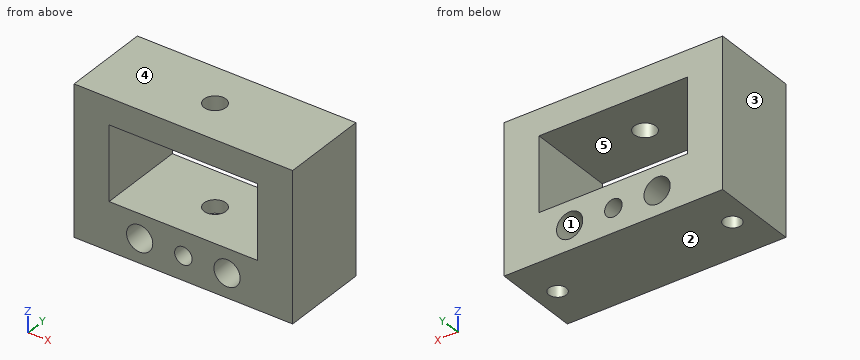
from build123d import *

# Parameters (mm, degrees)
SKETCH1_W                = 50
SKETCH1_H                = 20
BOSS_EXTRUDE1_DEPTH      = 11
SKETCH2_R                = 2
CUT_EXTRUDE1_DEPTH       = 11
SKETCH3_R                = 2
CUT_EXTRUDE2_DEPTH       = 21
SKETCH4_R                = 3
CUT_EXTRUDE3_DEPTH       = 21
SKETCH5_W                = 8
SKETCH5_H                = 20
BOSS_EXTRUDE2_DEPTH      = 22
SKETCH13_R               = 2.5
CUT_EXTRUDE6_DEPTH       = 3
SKETCH14_W               = 50
SKETCH14_H               = 20
BOSS_EXTRUDE4_DEPTH      = 1
BOSS_EXTRUDE4_DEPTH_BACK = 5
SKETCH15_R               = 2.5
CUT_EXTRUDE7_DEPTH       = 6
SKETCH18_R               = 2
CUT_EXTRUDE8_DEPTH       = 13


with BuildPart() as part:
    # Sketch1 → Boss-Extrude1 (new body)
    with BuildSketch(Plane.XY):
        Rectangle(SKETCH1_W, SKETCH1_H)
    extrude(amount=BOSS_EXTRUDE1_DEPTH)

    # Sketch2 → Cut-Extrude1 (cut)
    with BuildSketch(Plane(origin=(0, 0, 0), x_dir=(-1, 0, 0), z_dir=(0, 0, -1))):
        with Locations((-20, 0)):
            Circle(SKETCH2_R)
        with Locations((20, 0)):
            Circle(SKETCH2_R)
    extrude(amount=-CUT_EXTRUDE1_DEPTH, mode=Mode.SUBTRACT)

    # Sketch3 → Cut-Extrude2 (cut, through all)
    with BuildSketch(Plane.XZ.offset(10)):
        with Locations((0, 5.5)):
            Circle(SKETCH3_R)
    extrude(amount=-CUT_EXTRUDE2_DEPTH, mode=Mode.SUBTRACT)

    # Sketch4 → Cut-Extrude3 (cut, through all)
    with BuildSketch(Plane.XZ.offset(10)):
        with Locations((-10, 5.5)):
            Circle(SKETCH4_R)
        with Locations((10, 5.5)):
            Circle(SKETCH4_R)
    extrude(amount=-CUT_EXTRUDE3_DEPTH, mode=Mode.SUBTRACT)

    # Sketch5 → Boss-Extrude2 (add)
    with BuildSketch(Plane.XY.offset(11)):
        with Locations((-21, 0)):
            Rectangle(SKETCH5_W, SKETCH5_H)
        with Locations((21, 0)):
            Rectangle(SKETCH5_W, SKETCH5_H)
    extrude(amount=BOSS_EXTRUDE2_DEPTH)

    # Sketch13 → Cut-Extrude6 (cut)
    with BuildSketch(Plane.XY.offset(11)):
        Circle(SKETCH13_R)
    extrude(amount=-CUT_EXTRUDE6_DEPTH, mode=Mode.SUBTRACT)

    # Sketch14 → Boss-Extrude4 (add, two sides)
    with BuildSketch(Plane.XY.offset(33)) as boss_extrude4_sk:
        Rectangle(SKETCH14_W, SKETCH14_H)
    extrude(amount=BOSS_EXTRUDE4_DEPTH)
    extrude(boss_extrude4_sk.sketch, amount=-BOSS_EXTRUDE4_DEPTH_BACK)

    # Sketch15 → Cut-Extrude7 (cut)
    with BuildSketch(Plane.XY.offset(34)):
        Circle(SKETCH15_R)
    extrude(amount=-CUT_EXTRUDE7_DEPTH, mode=Mode.SUBTRACT)

    # Sketch18 → Cut-Extrude8 (cut)
    with BuildSketch(Plane(origin=(0, 0, 11), x_dir=(-1, 0, 0), z_dir=(0, 0, -1))):
        with Locations((-20, 0)):
            Circle(SKETCH18_R)
        with Locations((20, 0)):
            Circle(SKETCH18_R)
    extrude(amount=-CUT_EXTRUDE8_DEPTH, mode=Mode.SUBTRACT)


solid = part.part
Build history of the part. All positions in model axes, mm. Face numbers are marked on the shaded views. A direction names the side the tool comes from. Give positions to 0.01 mm unless a question says otherwise; leave off trailing zeros. Loops run counter-clockwise (first coordinate to the right, second up) from the corner with the lowest first, then second, coordinate; pieces in that order, holes last. Notation, with made-up numbers: (21.25, -9) -> (68.25, -9) arc R28 ccw to (68.25, 29) -> close; hole circle Ø8 at (41.5, 39.25). An arc over 180 degrees is marked (long way). Answer in a Markdown table with one row per item.
Item 1: Mould opens along X. For the marked faces 1, 2 and 3 say: pulls with the +X half, pulls with the -X half, needs draft (parallel to the pull), parting line crosses it, or undercut.
Findings below:
| item | result |
|---|---|
| face 1 | undercut |
| face 2 | needs draft |
| face 3 | pulls with the -X half |
Item 2: Slice it at B-B on x = 10. Write the cut outline in (y, z).
Findings below:
| item | result |
|---|---|
| outline | (-10, 0) -> (10, 0) -> (10, 2.5) -> (-10, 2.5) -> close; (-10, 8.5) -> (10, 8.5) -> (10, 11) -> (-10, 11) -> close; (-10, 28) -> (10, 28) -> (10, 34) -> (-10, 34) -> close |
Item 3: Slice it at A-A on z = 22.5. Write the cut outline in (x, y).
Findings below:
| item | result |
|---|---|
| outline | (-25, -10) -> (-17, -10) -> (-17, 10) -> (-25, 10) -> close; (17, -10) -> (25, -10) -> (25, 10) -> (17, 10) -> close; hole circle Ø4 at (-20, 0); hole circle Ø4 at (20, 0) |
Item 4: Slice it at C-C on z = 5.5. Write the cut outline in (x, y).
Findings below:
| item | result |
|---|---|
| outline | (-25, -10) -> (-13, -10) -> (-13, 10) -> (-25, 10) -> close; (-7, -10) -> (-2, -10) -> (-2, 10) -> (-7, 10) -> close; (2, -10) -> (7, -10) -> (7, 10) -> (2, 10) -> close; (13, -10) -> (25, -10) -> (25, 10) -> (13, 10) -> close; hole circle Ø4 at (-20, 0); hole circle Ø4 at (20, 0) |
Item 5: Probe line 1 along Z through (x, y) = (-10, -0.5); line 2 along Z through (x, y) = (0, 6.5); line 3 along Y through (x, z) = (20, 8). List the from-to ranges inside material, lowest first. Write a range as [from, to].
Findings below:
| item | result |
|---|---|
| line 1 | z = [0, 2.5], [8.5, 11], [28, 34] |
| line 2 | z = [0, 3.5], [7.5, 11], [28, 34] |
| line 3 | y = [-10, -2], [2, 10] |
Item 6: Flat gauge pins, fed straight in: P1, Ø1.5, axis at x = -1, y = -1, coming from the +Z side; P2, Ø3.5, axis at x = -20, y = 0, coming from the -Z side; P3, Ø3.5, axis at x = 10, z = 5.5, coming from the +Y side. Where does each tip first touch, or does it go through?
Findings below:
| item | result |
|---|---|
| P1 | stops at z = 8 |
| P2 | stops at z = 24 |
| P3 | passes through |
Item 7: Slice it at D-D on y = 8.25. Write the cut outline in (x, z).
Findings below:
| item | result |
|---|---|
| outline | (-25, 0) -> (25, 0) -> (25, 34) -> (-25, 34) -> close; hole (-17, 11) -> (17, 11) -> (17, 28) -> (-17, 28) -> close; hole circle Ø6 at (-10, 5.5); hole circle Ø4 at (0, 5.5); hole circle Ø6 at (10, 5.5) |
Item 8: Tool access for the marked faces 4 and 5: list every direction of +Z, -Z, +X, -X, +Y, -Y with a clear straight run to the whole face (end or side of a thin tool).
Findings below:
| item | result |
|---|---|
| face 4 | +Z, +X, -X, +Y, -Y |
| face 5 | +Y, -Y |
